Source: CAD feature listing. Evaluate the final solid. Frame: model axes, mm. Face numbers are marked on the shaded views. Give positions to 0.01 mm unless a question says otherwise; leave off trailing zeros. Write each loop counter-clockwise with the first axis right and the second up, starting at its lowest first coordinate (ties: lowest second). Pieces come first, ordered by that corner, then holes.
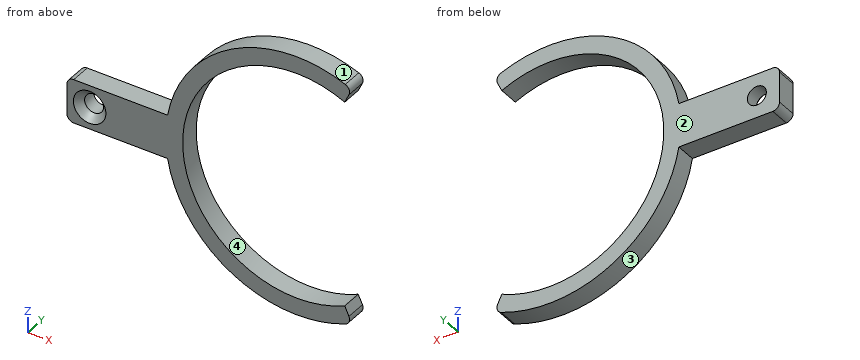
Autodesk Inventor part; units mm, degrees
ref_plane "YZ Plane" through (0, 0, 0) normal (1, 0, 0) x (0, 1, 0)
ref_plane "XZ Plane" through (0, 0, 0) normal (0, 1, 0) x (-1, 0, 0)
ref_plane "XY Plane" through (0, 0, 0) normal (0, 0, 1) x (1, 0, 0)
sketch "Sketch1" plane through (0, 0, 0) normal (0, 1, 0) x (-1, 0, 0)
  circle A0 centre (0, 0) radius 32.5
  line L0 (0, 32.5) -> (0, 102.5)
  line L1 (0, 102.5) -> (0, 169.7)
  circle A1 centre (0, 136.1) radius 33.6
  circle A2 centre (0, 136.1) radius 42.65
  line L2 (42.65, 136.1) -> (38.65, 136.1)
  line L3 (38.65, 136.1) -> (61.05, 136.1)
  circle A3 centre (61.05, 136.1) radius 22.4
  line L4 (61.05, 136.1) -> (61.05, 134.2)
  line L5 (61.05, 136.1) -> (61.05, 138)
  circle A4 centre (61.05, 136.1) radius 2.8
  line L6 (61.05, 138) -> (63.1067, 138)
  line L7 (61.05, 138) -> (58.9933, 138)
  line L8 (61.05, 134.2) -> (58.9933, 134.2)
  line L9 (61.05, 134.2) -> (63.1067, 134.2)
  circle A5 centre (61.05, 136.1) radius 4.7
  line L10 (0, -32.5) -> (0, -37.5)
  circle A6 centre (0, 0) radius 37.5
  line L11 (0, 32.5) -> (5, 32.5)
  line L12 (5, 32.5) -> (5, 93.7441)
  line L13 (0, 32.5) -> (-5, 32.5)
  line L14 (-5, 32.5) -> (-5, 93.7441)
  line L15 (0, 0) -> (29.257, 0) construction
  line L16 (0, 0) -> (37.5, 0) construction
  line L17 (0, 0) -> (32.476, 18.75)
  line L18 (0, 0) -> (37.5, 0) construction
  line L19 (0, 0) -> (-32.476, 18.75)
  line L20 (0, 0) -> (37.5, 0) construction
  line L21 (0, 169.7) -> (0, 174.7)
  circle A7 centre (0, 136.1) radius 38.6
  line L22 (65.75, 136.1) -> (67.75, 136.1)
  line L23 (62.4573, 140.5844) -> (62.4573, 142.5844)
  line L24 (62.4573, 131.6156) -> (62.4573, 129.6156)
  line L25 (5, 93.7441) -> (5, 102.8741)
  line L26 (-5, 93.7441) -> (-5, 102.8741)
  line L27 (62.4573, 129.6156) -> (32.9684, 129.6156)
  line L28 (62.4573, 142.5844) -> (32.9684, 142.5844)
  line L29 (62.4573, 142.5844) -> (67.75, 142.5844)
  line L30 (67.75, 142.5844) -> (67.75, 136.1)
  line L31 (67.75, 129.6156) -> (67.75, 136.1)
  line L32 (67.75, 129.6156) -> (62.4573, 129.6156)
  line L33 (0, 136.1) -> (-18.0247, 97.446)
  line L34 (0, 136.1) -> (42.65, 136.1) construction
  line L35 (0, 136.1) -> (-18.0247, 174.754)
  line L36 (0, 136.1) -> (42.65, 136.1) construction
  point P0 (37.3613, 126.4)
  point P1 (41.3134, 146.6937)
  point P2 (41.3134, 125.5063)
  point P3 (42.1542, 129.6156)
  point P4 (42.1542, 142.5844)
  point P5 (5, 97.8252)
  point P6 (38.0515, 129.6156)
  point P7 (39.6091, 129.6156)
  point P8 (39.6091, 142.5844)
  point P9 (38.0515, 142.5844)
  point P10 (-5, 97.8252)
  point P11 (-16.3131, 171.0835)
  point P12 (-14.2, 166.5519)
  point P13 (-14.2, 105.6481)
  point P14 (-16.3131, 101.1165)
  dimension "d0" = 65
  dimension "d1" = 70
  dimension "d2" = 67.2
  dimension "d3" = 85.3
  dimension "d4" = 4
  dimension "d6" = 22.4
  dimension "d7" = 1.9
  dimension "d8" = 1.9
  dimension "d9" = 5.6
  dimension "d10" = 9.4
  dimension "d11" = 5
  dimension "d12" = 5
  dimension "d13" = 5
  dimension "d16" = 30
  dimension "d17" = 150
  dimension "d18" = 5
  dimension "d19" = 2
  dimension "d20" = 2
  dimension "d21" = 2
  dimension "d28" = 115
  dimension "d29" = 115
extrude "Extrusion1" add sketch "Sketch1" along normal blind 6 contours A7 L26 A1 L0 | L0 A1 L25 A7 | A7 L33 A1 L26 | L25 A1 L27 A7 | L27 A3 L2 A2 | A2 L3 A5 L24 L27 | L27 A7 L28 A3 | L27 A1 L28 A7 | A7 L21 A1 L35 | L2 A3 L28 A2 | A2 L28 L23 A5 L3 | L24 A5 L22 L31 L32 | L21 A7 L28 A1 | A5 | L29 L30 L22 A5 L23
chamfer "Chamfer1" distance 2 angle 45 1 edges at (-58.25, 0, 136.1)
fillet "Fillet1" radius 2 4 edges at (-67.75, 3, 129.6156) (-67.75, 3, 142.5844) (16.3131, 3, 101.1165) (16.3131, 3, 171.0835)
properties part number "testing gear distances"
1. Cut plane A-A, the plane x = -61.05. Return the cut outline in (y, z), then the cut area to 3 significant figures.
2. Mould query, pull axis Z, two halves, no side actions, for the marked faces 1, 2, 3 and 4. Classes: +Z half, -Z half, draft (parallel to the pull), parting line (faces both ways), or undercut.
3. Cut plane C-C, the plane y = 4. Return the cut outline in (x, z), then the cut area to 3 significant figures.
4. Contact query for flat-ended pins moving along their axis: P1, Ø2, axis at y = 3.5, z = 128.5, coming from the +X side; P2, Ø1.8, axis at x = -45.5, y = 2, coming from the -Z side; P3, Ø2, axis at x = -7, y = 2.5, coming from the +Z side. Output: stop coordinate, or through.
5. Cut plane B-B, the plane z = 136.1. Return the cut outline in (x, y), then the cut area to 3 significant figures.
6. Line query: L1, parallel to X at y = 4.2, z = 136.1; L2, parallel to Z at x = -61.05, y = 3.75; L3, parallel to X at y = 1.55, z = 136.1. Output: solid intervals per line, ascending.
7. Cut plane D-D, the plane x = 0. Return the cut outline in (y, z), then the cut area to 3 significant figures.
Response values:
1. outline: (0, 129.62) - (6, 129.62) - (6, 133.3) - (2, 133.3) - (0, 131.3) - close; (0, 140.9) - (2, 138.9) - (6, 138.9) - (6, 142.58) - (0, 142.58) - close
1. area: 40.2 mm2
2. face 1: +Z half
2. face 2: draft
2. face 3: -Z half
2. face 4: undercut
3. outline: (-67.75, 131.62) arc R2 ccw to (-65.75, 129.62) - (-38.05, 129.62) arc R38.6 ccw to (14.38, 100.28) arc R2 ccw to (15.44, 102.98) - (14.2, 105.65) arc R33.6 cw (long way) to (14.2, 166.55) - (15.44, 169.22) arc R2 ccw to (14.38, 171.92) arc R38.6 ccw to (-38.05, 142.58) - (-65.75, 142.58) arc R2 ccw to (-67.75, 140.58) - close; hole circle Ø5.6 at (-61.05, 136.1)
3. area: 1,080 mm2
4. P1: stops at x = -32.48
4. P2: stops at z = 129.62
4. P3: stops at z = 174.23
5. outline: (-67.75, 0) - (-65.85, 0) - (-63.85, 2) - (-63.85, 6) - (-67.75, 6) - close; (-58.25, 2) - (-56.25, 0) - (-33.6, 0) - (-33.6, 6) - (-58.25, 6) - close
5. area: 167 mm2
6. L1: x = -67.75 to -63.85, -58.25 to -33.6
6. L2: z = 129.62 to 133.3, 138.9 to 142.58
6. L3: x = -67.75 to -64.3, -57.8 to -33.6
7. outline: (0, 97.5) - (6, 97.5) - (6, 102.5) - (0, 102.5) - close; (0, 169.7) - (6, 169.7) - (6, 174.7) - (0, 174.7) - close
7. area: 60.0 mm2
